Could you check a few things on this drawing? It's one solid part, dimensions in mm from its lowest x, y, z. A direction names the side the tool comes from. Give positions to 0.01 mm unless a question says otherwise; leave off trailing zeros. Order: outer loops, then holes, each group sorted by start corner. A loop starts at its lowest first (then second) coordinate and runs counter-clockwise, first axis right, second up. Notation, with made-up numbers: (25.25, -10.75) - (61.25, -10.75) arc R13 cw to (61.25, -0.75) - close; hole circle Ø8 at (-14, 56). An arc over 180 degrees is marked (long way). One line per question, with ' | ' between items. Start each with the question number.
1. If we mould it in two halves opening along Y, with no side actions, what happens to the marked faces 1, 2 and 3? For each: released by +Y, released by -Y, zero draft, split by the parting line, or undercut.
2. Which directions (+Z, -Z, +X, -X, +Y, -Y) give clear straight access to the entire face, cutting with the end or side of a thin tool? Please do the marked faces 4, 5 and 6.
3. Imagine slicing it at B-B (x = 17). Please give me the cut outline in (y, z), and give its area (3 significant figures).
4. I need wall thicknesses on probe 1 along Y at (x, z) = (4, 21); probe 2 along Z at (x, y) = (56.5, 21); probe 3 along X at (y, z) = (26.5, 69). Which ranges of each line are inside material? Lowest first, please. Write a range as from..to.
5. Imagine slicing it at A-A (z = 36). Please give me the cut outline in (x, y), and give its area (3 significant figures).
6. Imagine slicing it at C-C (y = 4.5). Please give me the cut outline in (x, z), and give its area (3 significant figures).
7. For P1, Ø5, axis at y = 23, z = 45.5, coming from the -X side; P2, Ø1.5, axis at y = 16, z = 42, coming from the +X side; P3, Ø6, axis at x = 9, y = 8, coming from the +Z side, each with a flat end and sliding along its axis, tell me the tip position at first contact or that it passes through.
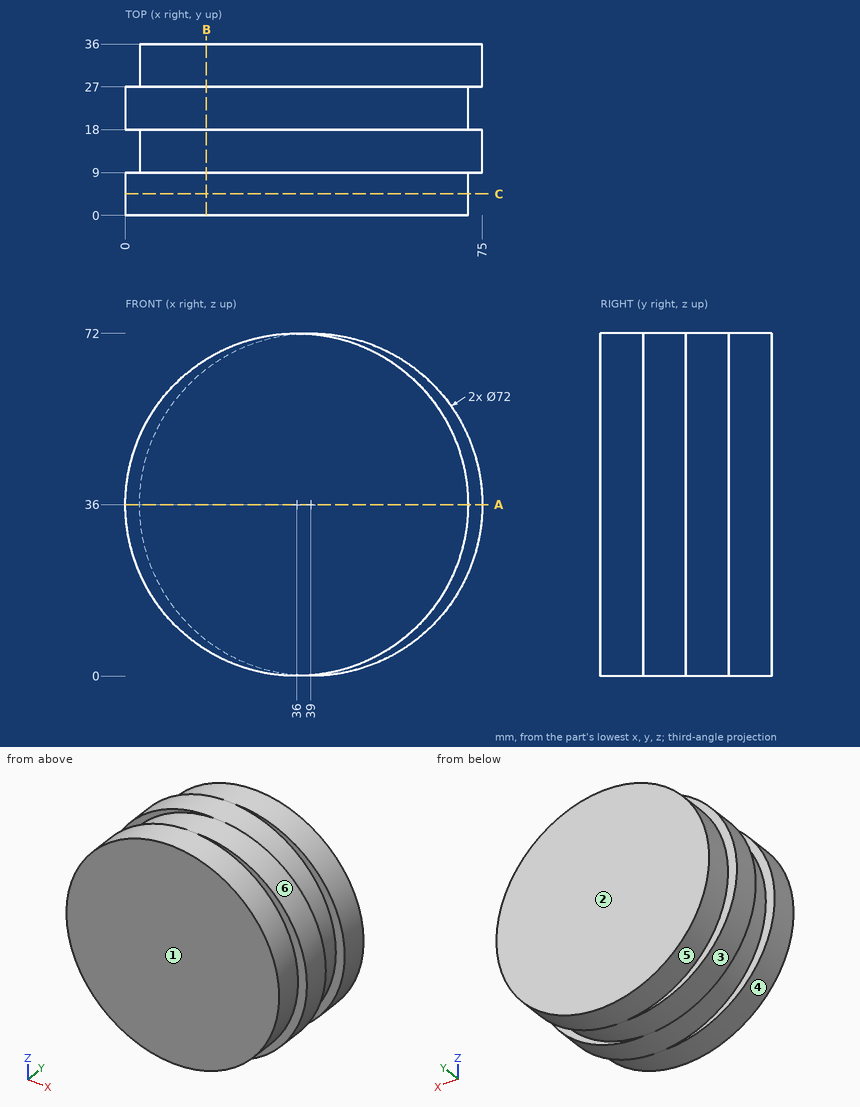
Results found:
1) face 1: released by -Y | face 2: released by +Y | face 3: undercut
2) face 4: -Y | face 5: +Y | face 6: none
3) outline: (0, 5.42) - (9, 5.42) - (9, 7.5) - (18, 7.5) - (18, 5.42) - (27, 5.42) - (27, 7.5) - (36, 7.5) - (36, 64.5) - (27, 64.5) - (27, 66.58) - (18, 66.58) - (18, 64.5) - (9, 64.5) - (9, 66.58) - (0, 66.58) - close | area: 2,130 mm2
4) probe 1: y = 0..9, 18..27 | probe 2: z = 6.41..65.59 | probe 3: x = 21.61..50.39
5) outline: (0, 0) - (72, 0) - (72, 9) - (75, 9) - (75, 18) - (72, 18) - (72, 27) - (75, 27) - (75, 36) - (3, 36) - (3, 27) - (0, 27) - (0, 18) - (3, 18) - (3, 9) - (0, 9) - close | area: 2,590 mm2
6) outline: circle Ø72 at (36, 36) | area: 4,070 mm2
7) P1: stops at x = 0.69 | P2: stops at x = 74.62 | P3: stops at z = 62.83
